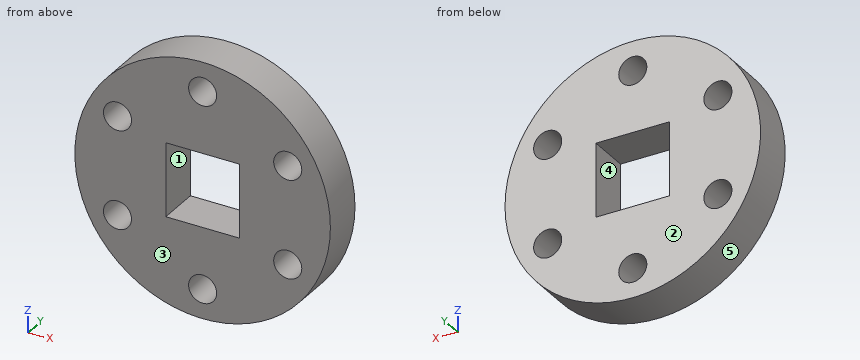
```python
from build123d import *

# Parameters (mm, degrees)
SKETCH1_R           = 18.2
BOSS_EXTRUDE1_DEPTH = 6
SKETCH2_R           = 2
CUT_EXTRUDE1_DEPTH  = 6
SKETCH3_W           = 10.5
SKETCH3_H           = 10.5
CUT_EXTRUDE2_DEPTH  = 6


with BuildPart() as part:
    # Sketch1 → Boss-Extrude1 (new body)
    with BuildSketch(Plane(origin=(0, 0, 0), x_dir=(1, 0, 0), z_dir=(0, 1, 0))):
        Circle(SKETCH1_R)
    extrude(amount=BOSS_EXTRUDE1_DEPTH)

    # Sketch2 → Cut-Extrude1 (cut)
    with BuildSketch(Plane(origin=(0, 6, 0), x_dir=(1, 0, 0), z_dir=(0, 1, 0))):
        with Locations((0, 14)):
            Circle(SKETCH2_R)
        with Locations((12.124355653, 7)):
            Circle(SKETCH2_R)
        with Locations((12.124355653, -7)):
            Circle(SKETCH2_R)
        with Locations((0, -14)):
            Circle(SKETCH2_R)
        with Locations((-12.124355653, -7)):
            Circle(SKETCH2_R)
        with Locations((-12.124355653, 7)):
            Circle(SKETCH2_R)
    extrude(amount=-CUT_EXTRUDE1_DEPTH, mode=Mode.SUBTRACT)

    # Sketch3 → Cut-Extrude2 (cut)
    with BuildSketch(Plane(origin=(0, 6, 0), x_dir=(1, 0, 0), z_dir=(0, 1, 0))):
        Rectangle(SKETCH3_W, SKETCH3_H)
    extrude(amount=-CUT_EXTRUDE2_DEPTH, mode=Mode.SUBTRACT)


solid = part.part
```
Check sheet for the modelled part. Datum: model origin and axes. Units: mm. Face numbers are marked on the shaded views. A direction names the side the tool comes from. Coordinates: 2 decimals unless noted, no trailing zeros. Write each loop counter-clockwise with the first axis right and the second up, starting at its lowest first coordinate (ties: lowest second). Pieces come first, ordered by that corner, then holes. Notation, with made-up numbers: M 8,31.25 L 64,31.25 A18 cw 64,44.25 Z; hole C 65,32 d5. An arc over 180 degrees is marked long. Write item = value, one per line. Start each with the question number.
1. Tool access check on the marked faces 1 and 2. Record the directions out of +Z, -Z, +X, -X, +Y, -Y that give a thin tool (end or side, any length) a straight path to the whole face; none if there is none.
2. Sectioned sample at D-D (x = -4.5). Record the cut outline in (y, z).
3. Thickness scan on probe 1 along Z at (x, y) = (0, 3.3); probe 2 along Z at (x, y) = (-11.5, 4.15); probe 3 along Z at (x, y) = (-10.5, 2.25). Record the ranges inside material, lowest first.
4. Go/stop test with flat-tipped pins: pin 1 (3 mm diameter, centred on y = 4, z = 12, fed in from +X); pin 2 (1.5 mm diameter, centred on x = -1.5, y = 3, fed in from +Z); pin 3 (5 mm diameter, centred on x = -12.12, z = -7, fed in from -Y); pin 4 (1.5 mm diameter, centred on x = -10.5, y = 4, fed in from +Z). Record where each tip stops, or that it passes through.
5. Sectioned sample at C-C (z = 0). Record the cut outline in (x, y).
6. Sectioned sample at A-A (z = 7). Record the cut outline in (x, y).
7. Mould release check, pull along Z, two halves, no side actions. Record for the marked faces 3, 4 and 5: pulls with the +Z half, pulls with the -Z half, needs draft (parallel to the pull), parting line crosses it, or undercut.
8. Sectioned sample at B-B (y = 1.6). Record the cut outline in (x, z).
The answers:
q1.face_1 = +Y, -Y
q1.face_2 = +Z, -Z, +X, -X, +Y
q2.outline = M 0,-17.63 L 6,-17.63 L 6,-5.25 L 0,-5.25 Z; M 0,5.25 L 6,5.25 L 6,17.63 L 0,17.63 Z
q3.probe_1 = -18.2 to -16, -12 to -5.25, 5.25 to 12, 16 to 18.2
q3.probe_2 = -14.11 to -8.9, -5.1 to 5.1, 8.9 to 14.11
q3.probe_3 = -14.87 to -8.17, -5.83 to 5.83, 8.17 to 14.87
q4.pin_1 = 14.87
q4.pin_2 = 18.18
q4.pin_3 = 0
q4.pin_4 = 15.37
q5.outline = M -18.2,0 L -5.25,0 L -5.25,6 L -18.2,6 Z; M 5.25,0 L 18.2,0 L 18.2,6 L 5.25,6 Z
q6.outline = M -16.8,0 L -14.12,0 L -14.12,6 L -16.8,6 Z; M -10.12,0 L 10.12,0 L 10.12,6 L -10.12,6 Z; M 14.12,0 L 16.8,0 L 16.8,6 L 14.12,6 Z
q7.face_3 = needs draft
q7.face_4 = undercut
q7.face_5 = parting line crosses it
q8.outline = C 0,0 d36.4; hole C -12.12,-7 d4; hole C -12.12,7 d4; hole M -5.25,-5.25 L 5.25,-5.25 L 5.25,5.25 L -5.25,5.25 Z; hole C 0,-14 d4; hole C 0,14 d4; hole C 12.12,-7 d4; hole C 12.12,7 d4
